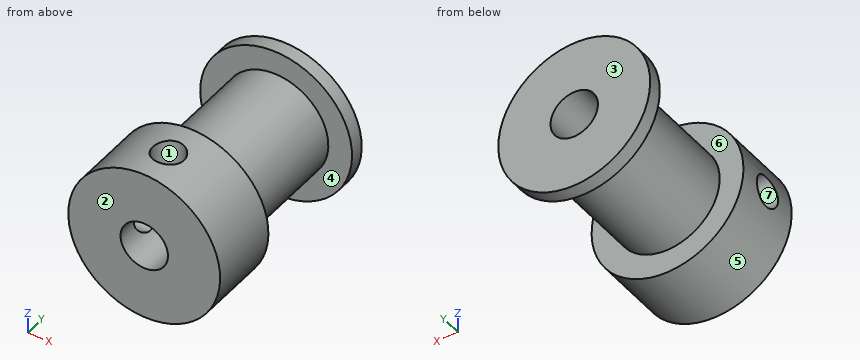
```python
from build123d import *

# Parameters (mm, degrees)
CROQUIS3_W     = 1.65
CROQUIS3_H     = 8.001
MATRIZC1_COUNT = 2
MATRIZC1_ANGLE = 90


with BuildPart() as part:
    # Croquis1 → Revolución1 (revolve)
    with BuildSketch(Plane.XY, mode=Mode.PRIVATE) as revoluci_n1_sk:
        Polygon((8, 7.5), (8, 0), (2.5, 0), (2.5, 22), (8, 22), (8, 20.5), (5.5, 20.5), (5.5, 7.5), align=None)
    revolve(revoluci_n1_sk.sketch.rotate(Axis((0, 0, 0), (0, 1, 0)), 90), axis=Axis((0, 0, 0), (0, 1, 0)))

    # Croquis3 → Taladro roscado M41 (revolve, cut)
    with BuildSketch(Plane(origin=(0, 3.75, 0), x_dir=(0, 1, 0), z_dir=(1, 0, 0))):
        with Locations((0.825, 4.0005)):
            Rectangle(CROQUIS3_W, CROQUIS3_H)
    taladro_roscado_m41 = revolve(axis=Axis((0, 3.75, -6.35), (0, 0, 1)), mode=Mode.SUBTRACT)

    # MatrizC1: Taladro roscado M41 ×2 about axis
    matrizc1_axis = Axis((0, 0, 0), (0, -1, 0))
    for i in range(1, MATRIZC1_COUNT):
        add(taladro_roscado_m41.rotate(matrizc1_axis, i * MATRIZC1_ANGLE / (MATRIZC1_COUNT - 1)), mode=Mode.SUBTRACT)


solid = part.part
```
Geometry check sheet. Reference: the model listing, model coordinates, mm. Face numbers are marked on the shaded views. A direction names the side the tool comes from. Round coordinates to 2 decimals unless told otherwise and drop trailing zeros. Order: outer loops, then holes, each group sorted by start corner. A loop starts at its lowest first (then second) coordinate and runs counter-clockwise, first axis right, second up. Notation, with made-up numbers: (-11, 88) - (8, 88) arc R16 ccw to (8, 108) - close; hole circle Ø9 at (73.5, 78.25). An arc over 180 degrees is marked (long way). Use a Markdown table: item, result. Add a question column.
(1) Release check for a two-part mould opening along Y. For the marked faces 1, 2, 3 and 4 record: pulls with the +Y half, pulls with the -Y half, needs draft (parallel to the pull), parting line crosses it, or undercut.
(2) Sectioned sample at D-D, the plane y = 7. Enter the section's corners in (x, z), and give its area (3 significant figures).
(3) Sectioned sample at B-B, the plane z = 0. Enter the section's corners in (x, y).
(4) Sectioned sample at C-C, the plane y = 4. Enter the section's corners in (x, z), and give its area (3 significant figures).
(5) Depth check by flat-ended pin: pin 1 (8 mm diameter, centred on x = -0.5, z = -0.5, fed in from +Y); pin 2 (1 mm diameter, centred on x = -5.5, y = 13, fed in from +Z); pin 3 (2 mm diameter, centred on x = -0.5, y = 9.5, fed in from +Z); pin 4 (8 mm diameter, centred on x = -6, y = 14.5, fed in from +Z). Enter the tip coordinate at first touch or a pass-through.
(6) Material ranges on line 1 along Y through (x, z) = (0, 6); line 2 along Y through (x, z) = (5.5, 4.75); line 3 along Y through (x, z) = (0, 3.5), recorded low to high. Write a range as [from, to].
(7) Sectioned sample at A-A, the plane x = 0. Enter the section's corners in (y, z), and give its area (3 significant figures).
(8) Tool access check on the marked faces 5, 6 and 7. Record the directions out of +Z, -Z, +X, -X, +Y, -Y that give a thin tool (end or side, any length) a straight path to the whole face; none if there is none.
Answers below:
| question | item | result |
|---|---|---|
| 1 | face 1 | undercut |
| 1 | face 2 | pulls with the -Y half |
| 1 | face 3 | pulls with the +Y half |
| 1 | face 4 | undercut |
| 2 | outline | circle Ø16 at (0, 0); hole circle Ø5 at (0, 0) |
| 2 | area | 181 mm² |
| 3 | outline | (-8, 0) - (-2.5, 0) - (-2.5, 2.1) - (-8, 2.1) - close; (-8, 5.4) - (-2.5, 5.4) - (-2.5, 22) - (-8, 22) - (-8, 20.5) - (-5.5, 20.5) - (-5.5, 7.5) - (-8, 7.5) - close; (2.5, 0) - (8, 0) - (8, 7.5) - (5.5, 7.5) - (5.5, 20.5) - (8, 20.5) - (8, 22) - (2.5, 22) - close |
| 4 | outline | (-7.83, -1.63) arc R8 ccw (long way) to (1.63, 7.83) - (1.63, 1.89) arc R2.5 cw (long way) to (-1.89, -1.63) - close; (-7.83, 1.63) - (-1.89, 1.63) arc R2.5 cw to (-1.63, 1.89) - (-1.63, 7.83) arc R8 ccw to start |
| 4 | area | 145 mm² |
| 5 | pin 1 | y = 22 |
| 5 | pin 2 | z = 2.29 |
| 5 | pin 3 | z = 5.5 |
| 5 | pin 4 | z = 5.12 |
| 6 | line 1 | [0, 2.1], [5.4, 7.5], [20.5, 22] |
| 6 | line 2 | [0, 7.5], [20.5, 22] |
| 6 | line 3 | [0, 2.1], [5.4, 22] |
| 7 | outline | (0, -8) - (7.5, -8) - (7.5, -5.5) - (20.5, -5.5) - (20.5, -8) - (22, -8) - (22, -2.5) - (0, -2.5) - close; (0, 2.5) - (2.1, 2.5) - (2.1, 8) - (0, 8) - close; (5.4, 2.5) - (22, 2.5) - (22, 8) - (20.5, 8) - (20.5, 5.5) - (7.5, 5.5) - (7.5, 8) - (5.4, 8) - close |
| 7 | area | 159 mm² |
| 8 | face 5 | +Y, -Y |
| 8 | face 6 | none |
| 8 | face 7 | -X |
